Input: dimensioned drawing with shaded views. Units: mm. Origin: part minimum x, y, z. A direction names the side the tool comes from. Give positions to 0.01 mm unless a question says otherwise; leave off trailing zeros. Write each loop counter-clockwise with the first axis right and the second up, starting at its lowest first coordinate (ties: lowest second). Pieces come first, ordered by that corner, then holes. Notation, with made-up numbers: M 80.25,28.25 L 94.25,28.25 A31 cw 94.25,65.25 Z; hole C 32,60.5 d10. An arc over 180 degrees is marked long. Answer as a JSON object with one key per item and string values.
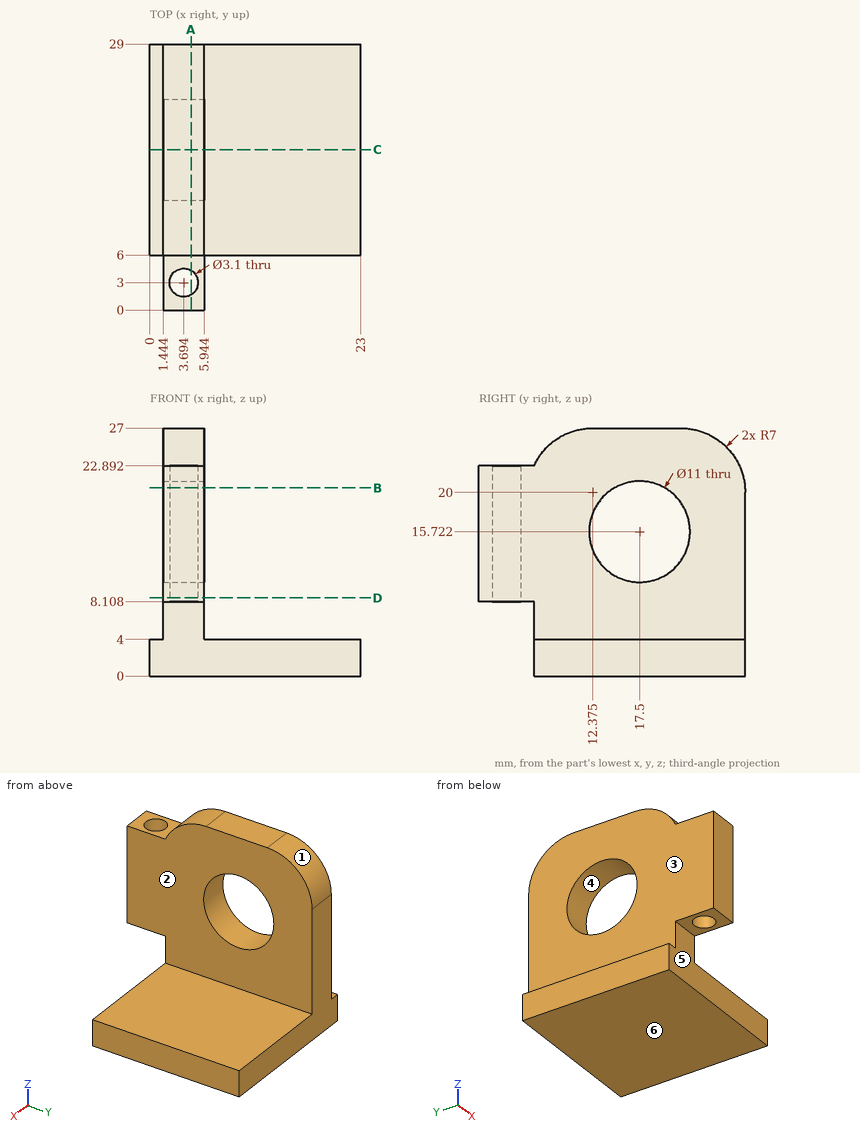
1) Cut plane C-C on y = 17.5. Return loops of the section in (x, z), and give its area (3 significant figures).
Geometry check:
{"outline": "M 0,0 L 23,0 L 23,4 L 5.94,4 L 5.94,10.22 L 1.44,10.22 L 1.44,4 L 0,4 Z; M 1.44,21.22 L 5.94,21.22 L 5.94,27 L 1.44,27 Z", "area": "146 mm2"}
2) Cut plane D-D on z = 8.5. Return loops of the section in (x, y).
Geometry check:
{"outline": "M 1.44,0 L 5.94,0 L 5.94,29 L 1.44,29 Z; hole C 3.69,3 d3.1"}
3) Set-up query: the marked faces 1, 2 and 3. Return all of +Z, -Z, +X, -X, +Y, -Y with unobstructed straight access to the full face (end or side cutting, diameter ignored); none if empty.
Geometry check:
{"face 1": "+Z, +X, -X, +Y", "face 2": "+Z, +X, +Y, -Y", "face 3": "+Z, -X, +Y, -Y"}
4) Line query: line 1 (Z direction, x = 3.1, y = 17.5); line 2 (X direction, y = 8.5, z = 5); line 3 (Z direction, x = 20.5, y = 25). Output: solid intervals per line, ascending. Write a range as from..to.
Geometry check:
{"line 1": "z = 0..10.22, 21.22..27", "line 2": "x = 1.44..5.94", "line 3": "z = 0..4"}
5) Contact query for flat-ended pins moving along their axis: P1, Ø7, axis at y = 12.5, z = 17, coming from the +X side; P2, Ø5, axis at x = 3, y = 3, coming from the -Z side; P3, Ø5, axis at y = 12, z = 20, coming from the -X side. Output: stop coordinate, or through.
Geometry check:
{"P1": "stops at x = 5.94", "P2": "stops at z = 8.11", "P3": "stops at x = 1.44"}
6) Pull-direction query (Z, two-part tool) for the marked faces 4, 5 and 6; classes: pulls with the +Z half, pulls with the -Z half, needs draft (parallel to the pull), parting line crosses it, or undercut.
Geometry check:
{"face 4": "undercut", "face 5": "needs draft", "face 6": "pulls with the -Z half"}
7) Cut plane A-A on x = 4.5. Return loops of the section in (y, z) (1 decimal), and give its area (3 significant figures).
Geometry check:
{"outline": "M 0,8.1 L 1.7,8.1 L 1.7,22.9 L 0,22.9 Z; M 4.3,8.1 L 6,8.1 L 6,0 L 29,0 L 29,20 A7 ccw 22,27 L 12.4,27 A7 ccw 6,22.9 L 4.3,22.9 Z; hole C 17.5,15.7 d11", "area": "558 mm2"}
8) Cut plane B-B on z = 20.5. Return loops of the section in (x, y).
Geometry check:
{"outline": "M 1.44,0 L 5.94,0 L 5.94,14.78 L 1.44,14.78 Z; M 1.44,20.22 L 5.94,20.22 L 5.94,28.98 L 1.44,28.98 Z; hole C 3.69,3 d3.1"}
